Source: three-view drawing plus pictorial views. Frame: mm from the lowest corner of the part. A direction names the side the tool comes from. Give positions to 0.01 mm unless a question says otherwise; leave off trailing zeros. Loops run counter-clockwise (first coordinate to the right, second up) from the corner with the lowest first, then second, coordinate; pieces in that order, holes last. Notation, with made-up numbers: M -6.75,-13 L 38.25,-13 A19 ccw 38.25,10 Z; hole C 3,8.5 d8. An arc over 180 degrees is marked long. One line per item, written item: value. Start each with the question number.
(1) Section C-C on z = 10.75. Output: boundary loops of the cut face in (x, y) (3 decimals).
(2) Ray query, line 1 along Y through (x, z) = (12.5, 11); line 2 along Y through (x, z) = (14, 11.75) (3 decimals); line 3 along X through (y, z) = (20, 4). Return the intervals inside material, ascending. Write a range as from..to.
(3) Section B-B on y = 12.5. Output: boundary loops of the cut face in (x, z).
(4) Pull-direction query (Y, two-part tool) for the marked faces 1, 2 and 3; classes: released by +Y, released by -Y, zero draft, split by the parting line, or undercut.
(5) Access query for the marked faces 4 and 5. Directions: +Z, -Z, +X, -X, +Y, -Y. A direction counts if a zero-diameter tool reaches every point of the face in a straight line with its end or side. Return the directions, or none.
(6) Pin query (flat end, axial travel): P1, Ø6, axis at x = 8, z = 4, coming from the -Y side; P2, Ø6, axis at x = 16.5, z = 10, coming from the +Y side; P3, Ø1.7, axis at x = 12.5, y = 20, coming from the -Z side; P4, Ø4.5, axis at y = 8, z = 8, coming from the +X side. Return the tip coordinate at first contact, or that it passes through.
(7) Section A-A on x = 5. Output: boundary loops of the cut face in (y, z).
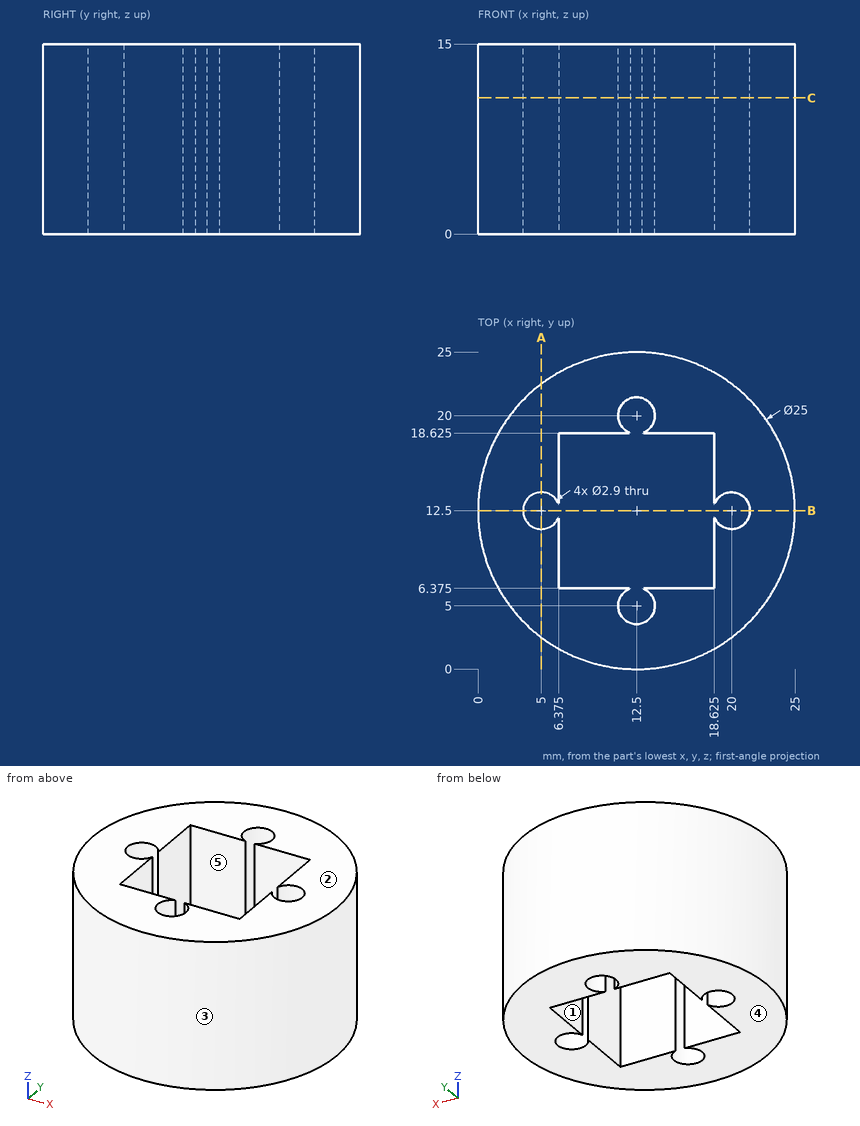
Output values:
1. outline: C 12.5,12.5 d25; hole M 6.375,6.375 L 12.04,6.375 A1.45 ccw long 12.96,6.375 L 18.625,6.375 L 18.625,12.04 A1.45 ccw long 18.625,12.96 L 18.625,18.625 L 12.96,18.625 A1.45 ccw long 12.04,18.625 L 6.375,18.625 L 6.375,12.96 A1.45 ccw long 6.375,12.04 Z
2. line 1: y = 0..3.55, 21.45..25
2. line 2: y = 0.09..6.375, 18.625..24.91
2. line 3: x = 2.5..11.05, 13.95..22.5
3. outline: M 0,0 L 3.55,0 L 3.55,15 L 0,15 Z; M 21.45,0 L 25,0 L 25,15 L 21.45,15 Z
4. face 1: undercut
4. face 2: zero draft
4. face 3: split by the parting line
5. face 4: -Z, +X, -X, +Y, -Y
5. face 5: +Z, -Z
6. P1: stops at y = 0.09
6. P2: stops at y = 24.96
6. P3: passes through
6. P4: stops at x = 24.8
7. outline: M 2.5,0 L 11.05,0 L 11.05,15 L 2.5,15 Z; M 13.95,0 L 22.5,0 L 22.5,15 L 13.95,15 Z
